Build history of the part. All positions in model axes, mm. Face numbers are marked on the shaded views. A direction names the side the tool comes from. Give positions to 0.01 mm unless a question says otherwise; leave off trailing zeros. Write each loop counter-clockwise with the first axis right and the second up, starting at its lowest first coordinate (ties: lowest second). Pieces come first, ordered by that corner, then holes. Notation, with made-up numbers: M 81.25,-36 L 117.25,-36 A24 cw 117.25,-2 Z; hole C -36,-25 d6. An arc over 180 degrees is marked long. One line per item, written item: value. Start each with the question number.
from build123d import *

# Parameters (mm, degrees)
SKETCH1_W           = 18
SKETCH1_H           = 15
BOSS_EXTRUDE1_DEPTH = 35
SKETCH2_R           = 5
CUT_EXTRUDE1_DEPTH  = 16
SKETCH3_R           = 3
CUT_EXTRUDE2_DEPTH  = 8


with BuildPart() as part:
    # Sketch1 → Boss-Extrude1 (new body)
    with BuildSketch(Plane(origin=(0, 0, 0), x_dir=(0, 0, -1), z_dir=(1, 0, 0))):
        with Locations((-18.782608696, 5.413043478)):
            Rectangle(SKETCH1_W, SKETCH1_H)
    extrude(amount=BOSS_EXTRUDE1_DEPTH)

    # Sketch2 → Cut-Extrude1 (cut, through all)
    with BuildSketch(Plane(origin=(0, -2.086956522, 0), x_dir=(-1, 0, 0), z_dir=(0, -1, 0))):
        with Locations((-27, -18.782608696)):
            Circle(SKETCH2_R)
    extrude(amount=-CUT_EXTRUDE1_DEPTH, mode=Mode.SUBTRACT)

    # Sketch3 → Cut-Extrude2 (cut)
    with BuildSketch(Plane.ZY):
        with Locations((18.782608696, 5.413043478)):
            Circle(SKETCH3_R)
    extrude(amount=-CUT_EXTRUDE2_DEPTH, mode=Mode.SUBTRACT)


solid = part.part
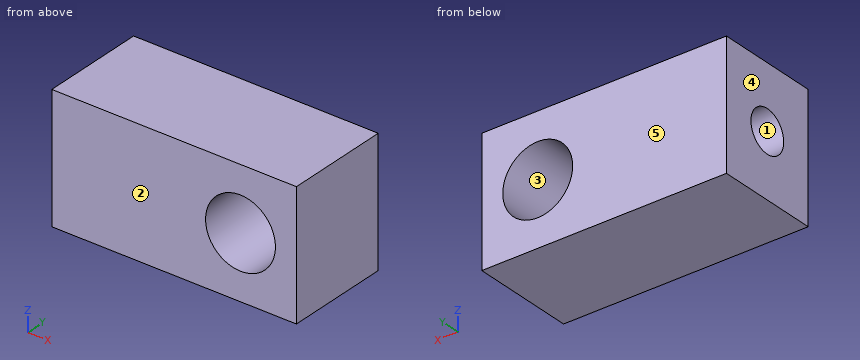
1) Band-saw the part on C-C (y = 2.75). List the corners of the cut face in (x, z).
2) Probe line 1 along X through (y, z) = (12, 18.75); line 2 along X through (y, z) = (8.75, 20.5); line 3 along Z through (x, y) = (26, 8). List the from-to ranges inside material, lowest first. Write a range as from..to.
3) Band-saw the part on A-A (x = 27). List the corners of the cut face in (y, z).
4) Band-saw the part on D-D (z = 15.25). List the corners of the cut face in (x, y), then the cut area to 3 significant figures.
5) Mould opens along X. For the marked faces 3, 4 and 5 say: released by +X, released by -X, zero draft, split by the parting line, or undercut.
6) Band-saw the part on B-B (z = 21). List the corners of the cut face in (x, y).
7) Tool access for the marked faces 1 and 2: list every direction of +Z, -Z, +X, -X, +Y, -Y with a clear straight run to the whole face (end or side of a thin tool).
8) Drop flat-ended pins along their axis: P1, Ø3.5, axis at y = 5.41, z = 18.78, coming from the -X side; P2, Ø3, axis at y = 3, z = 24.5, coming from the -X side. Give the stop position or say it passes through.
Model answer:
1. outline: M 0,9.78 L 35,9.78 L 35,27.78 L 0,27.78 L 0,20.16 L 8,20.16 L 8,17.4 L 0,17.4 Z; hole C 27,18.78 d10
2. line 1: x = 0..22, 32..35
2. line 2: x = 0..22.3, 31.7..35
2. line 3: z = 9.78..13.88, 23.68..27.78
3. outline: M -2.09,9.78 L 12.91,9.78 L 12.91,13.78 L -2.09,13.78 Z; M -2.09,23.78 L 12.91,23.78 L 12.91,27.78 L -2.09,27.78 Z
4. outline: M 0,-2.09 L 23.46,-2.09 L 23.46,12.91 L 0,12.91 Z; M 30.54,-2.09 L 35,-2.09 L 35,12.91 L 30.54,12.91 Z
4. area: 419 mm²
5. face 3: undercut
5. face 4: released by -X
5. face 5: zero draft
6. outline: M 0,-2.09 L 22.52,-2.09 L 22.52,12.91 L 0,12.91 L 0,7.43 L 8,7.43 L 8,3.39 L 0,3.39 Z; M 31.48,-2.09 L 35,-2.09 L 35,12.91 L 31.48,12.91 Z
7. face 1: -X
7. face 2: +Z, -Z, +X, -X, -Y
8. P1: stops at x = 8
8. P2: stops at x = 0
